```python
from build123d import *

# Parameters (mm, degrees)
F0_W     = 584.2
F0_H     = 438.15
F1_DEPTH = 9.525
F2_W     = 6.35
F2_H     = 876.3
F3_DEPTH = 12.7
F4_W     = 584.2
F4_H     = 19.05
F5_DEPTH = 6.35
F6_W     = 76.2
F6_H     = 101.6
F7_DEPTH = 19.051


with BuildPart() as f1:
    # F0 (on Front) → F1 (new body, symmetric)
    with BuildSketch(Plane.XZ):
        with Locations((44.1960046741, 219.075)):
            Rectangle(F0_W, F0_H)
        with Locations((44.1960046741, -219.075)):
            Rectangle(F0_W, F0_H)
    extrude(amount=F1_DEPTH, both=True)

    # F2 (on face) → F3 (cut)
    with BuildSketch(Plane(origin=(0, 9.525, 0), x_dir=(-1, 0, 0), z_dir=(0, 1, 0))):
        with Locations((-333.1210046741, 0)):
            Rectangle(F2_W, F2_H)
        with Locations((244.7289953259, 0)):
            Rectangle(F2_W, F2_H)
    extrude(amount=-F3_DEPTH, mode=Mode.SUBTRACT)

    # F4 (on face) → F5 (cut)
    with BuildSketch(Plane(origin=(0, 9.525, 0), x_dir=(-1, 0, 0), z_dir=(0, 1, 0))):
        with Locations((-44.1960046741, 309.5625)):
            Rectangle(F4_W, F4_H)
    extrude(amount=-F5_DEPTH, mode=Mode.SUBTRACT)

    # F6 (on face) → F7 (cut, through all)
    with BuildSketch(Plane.XZ.offset(9.525)):
        with Locations((-209.8039953259, 387.35)):
            Rectangle(F6_W, F6_H)
    extrude(amount=-F7_DEPTH, mode=Mode.SUBTRACT)


solid = f1.part
```
The listing builds one solid part. Answer for the finished solid, in the listing's coordinates (mm). A direction names the side the tool comes from. Round coordinates to 2 decimals unless told otherwise and drop trailing zeros. Loops run counter-clockwise (first coordinate to the right, second up) from the corner with the lowest first, then second, coordinate; pieces in that order, holes last. Notation, with made-up numbers: (85, 21) - (108, 21) arc R19 cw to (108, 33) - close; hole circle Ø11 at (-7.5, -28.5). An arc over 180 degrees is marked (long way). Use one line per item in the form item = value. Start each with the question number.
1. Consider line 1 (Z direction, x = 14, y = 7.5); line 2 (X direction, y = -2.25, z = -95); line 3 (X direction, y = 0, z = 340.5). Determine where each line is inside the solid, lowest interval first. Write a range as [from, to].
2. The part is cut by section A-A on y = 0. Determine the outline of the cut face in (x, z).
3. Given pin 1 Ø9.5 at (y, z) = (-4, 388.5) entering from -X; pin 2 Ø7 at (x, z) = (-246, -98) entering from +Y (3 decimals); pin 3 Ø6 at (y, z) = (0.5, 85.5) entering from -X, each flat-ended and moving along its own axis, determine where each tip first touches the part or whether it passes through.
4. A tool of negligible diameter and unlimited length cuts with its end or side. For faces 1 (the face through (-171.704, 0, 387)), 2 (the face through (48, 3.175, 310)), 3 (the face through (40, -9.525, 6)), from which of +Z, -Z, +X, -X, +Y, -Y can it reach the whole face along a straight path? Write none if from no direction.
Geometry check:
q1.line_1 = [-438.15, 300.04], [319.09, 438.15]
q1.line_2 = [-241.55, 329.95]
q1.line_3 = [-171.7, 329.95]
q2.outline = (-241.55, -438.15) - (329.95, -438.15) - (329.95, 438.15) - (-171.7, 438.15) - (-171.7, 336.55) - (-241.55, 336.55) - close
q3.pin_1 = -171.7
q3.pin_2 = -3.175
q3.pin_3 = -241.55
q4.face_1 = +Z, -X, +Y, -Y
q4.face_2 = +X, -X, +Y
q4.face_3 = +Z, -Z, +X, -X, -Y
